Read the model definition and answer for the solid it produces. Units are mm, in the model's axes. Give positions to 0.01 mm unless a question says otherwise; leave off trailing zeros. Write each loop counter-clockwise with the first axis right and the second up, starting at its lowest first coordinate (ties: lowest second). Pieces come first, ordered by that corner, then holes. Notation, with made-up numbers: (66.5, 48.5) - (98.5, 48.5) arc R33 ccw to (98.5, 86.5) - close; hole circle Ø11 at (3.25, -6.5). An arc over 180 degrees is marked (long way). Answer as CSV lines item,"result".
Solid Edge part; units mm, degrees
sketch "Sketch1" plane through (0, 0, 0) normal (0, -1, 0) x (1, 0, 0)
  line L0 (15, 66.9946) -> (15, 6.9946)
  line L1 (15, 6.9946) -> (0, 0)
  line L2 (0, 0) -> (-15, 6.9946)
  line L3 (-15, 6.9946) -> (-15, 66.9946)
  line L4 (-15, 66.9946) -> (15, 66.9946)
extrude "Protrusion1" add sketch "Sketch1" against normal blind 400
sketch "Sketch2" plane through (15, 35, 21.0229) normal (1, 0, 0) x (0, 1, 0)
  line L0 (365, 45.9717) -> (308.7848, -21.0229)
  line L1 (308.7848, -21.0229) -> (365, -21.0229)
  line L2 (365, -21.0229) -> (365, 45.9717)
extrude "Cutout1" cut sketch "Sketch2" against normal up to next
properties material "ABS 20% Infill"
(1) A cutting plane is placed at A-A (y = 251). Write down the section's boundary in (x, z).
Worked out:
outline,"(-15, 6.99) - (0, 0) - (15, 6.99) - (15, 66.99) - (-15, 66.99) - close"
(2) Find the intervals of material crossed by L1, parallel to Y at x = 1.5, z = 15; L2, parallel to Z at x = 11.5, y = 177.5; L3, parallel to Z at x = 1, y = 219, in increasing order.
Worked out:
L1,"y = 0 to 356.37"
L2,"z = 5.36 to 66.99"
L3,"z = 0.47 to 66.99"
(3) Each of these flat-tipped pins is pushed along its axis until it touches: P1, Ø2, axis at x = -3, z = 21, coming from the +Y side (3 decimals); P2, Ø1, axis at x = -11, z = 51.5, coming from the -Y side. Where does it stop, or does it pass through?
Worked out:
P1,"stops at y = 362.245"
P2,"stops at y = 0"
(4) A cutting plane is placed at B-B (x = -7). Write down the section's boundary in (y, z), and give its area (3 significant figures).
Worked out:
outline,"(0, 3.26) - (346.52, 3.26) - (400, 66.99) - (0, 66.99) - close"
area,"23,800 mm^2"
(5) A cutting plane is placed at C-C (z = 43). Write down the section's boundary in (x, y), and give its area (3 significant figures).
Worked out:
outline,"(-15, 0) - (15, 0) - (15, 379.87) - (-15, 379.87) - close"
area,"11,400 mm^2"
